Verification items for the finished model (mm, model axes). Give positions to 0.01 mm unless a question says otherwise; leave off trailing zeros. Loops run counter-clockwise (first coordinate to the right, second up) from the corner with the lowest first, then second, coordinate; pieces in that order, holes last. Notation, with made-up numbers: M 55.25,45 L 65.25,45 A28 ccw 65.25,64 Z; hole C 63,52 d9. An arc over 180 degrees is marked long. Answer in a Markdown table with one row per item.
```python
from build123d import *

# Parameters (mm, degrees)
MASTER_SKETCH_WING_GEOMETRY_MASTER_SKETC_W   = 92
MASTER_SKETCH_WING_GEOMETRY_MASTER_SKETC_H   = 38
MASTER_SKETCH_WING_GEOMETRY_MASTER_SKETC_W_2 = 82
MASTER_SKETCH_WING_GEOMETRY_MASTER_SKETC_H_2 = 28
BOSS_EXTRUDE2_DEPTH                          = 841


with BuildPart() as part:
    # Master sketch-Wing Geometry Master Sketc → Boss-Extrude2 (new body)
    with BuildSketch(Plane.XY):
        with Locations((90.000000001, 9.799999997)):
            Rectangle(MASTER_SKETCH_WING_GEOMETRY_MASTER_SKETC_W, MASTER_SKETCH_WING_GEOMETRY_MASTER_SKETC_H)
        with Locations((90.000000001, 9.799999997)):
            Rectangle(MASTER_SKETCH_WING_GEOMETRY_MASTER_SKETC_W_2, MASTER_SKETCH_WING_GEOMETRY_MASTER_SKETC_H_2, mode=Mode.SUBTRACT)
    extrude(amount=BOSS_EXTRUDE2_DEPTH)


solid = part.part
```
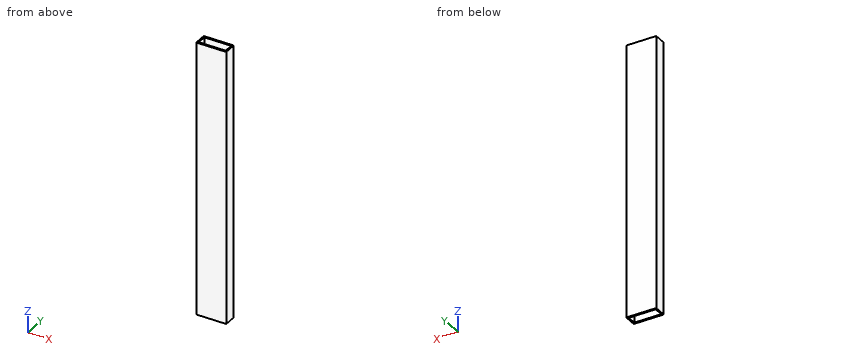
Item 1: Sectioned sample at C-C (z = 117). Record the cut outline in (x, y), and give its area (3 significant figures).
Reported:
| item | result |
|---|---|
| outline | M 44,-9.2 L 136,-9.2 L 136,28.8 L 44,28.8 Z; hole M 49,-4.2 L 131,-4.2 L 131,23.8 L 49,23.8 Z |
| area | 1,200 mm^2 |
Item 2: Sectioned sample at A-A (y = 2.5). Record the cut outline in (x, z).
Reported:
| item | result |
|---|---|
| outline | M 44,0 L 49,0 L 49,841 L 44,841 Z; M 131,0 L 136,0 L 136,841 L 131,841 Z |
Item 3: Scan lines: L1, parallel to Y at x = 127.5, z = 539.5; L2, parallel to X at y = 11.5, z = 115. Record each from-to range of solid material in increasing order. Write a range as [from, to].
Reported:
| item | result |
|---|---|
| L1 | y = [-9.2, -4.2], [23.8, 28.8] |
| L2 | x = [44, 49], [131, 136] |
Item 4: Sectioned sample at B-B (x = 98). Record the cut outline in (y, z), and give its area (3 significant figures).
Reported:
| item | result |
|---|---|
| outline | M -9.2,0 L -4.2,0 L -4.2,841 L -9.2,841 Z; M 23.8,0 L 28.8,0 L 28.8,841 L 23.8,841 Z |
| area | 8,410 mm^2 |
